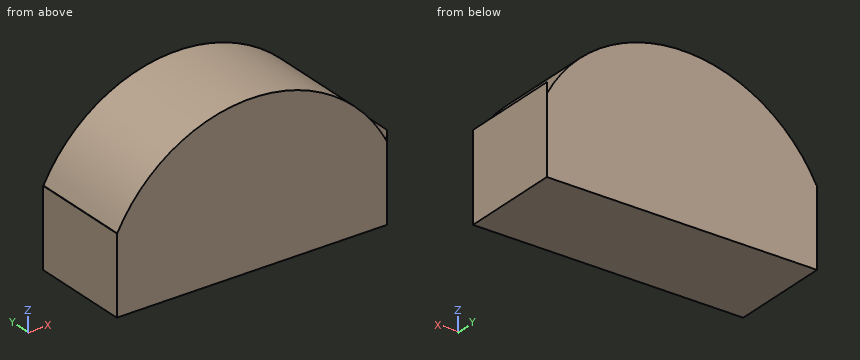
Solid Edge part; units mm, degrees
sketch "Sketch1" plane through (0, 0, 0) normal (0, 0, 1) x (1, 0, 0)
  line L0 (-40, -15) -> (40, -15)
  line L1 (40, -15) -> (40, 15)
  line L2 (40, 15) -> (-40, 15)
  line L3 (-40, 15) -> (-40, -15)
extrude "Protrusion1" add sketch "Sketch1" against normal blind 47
sketch "Sketch2" plane through (0, -15, -23.5) normal (0, -1, 0) x (1, 0, 0)
  arc A0 (39.8736, -0.641) -> (-39.8736, -0.641) centre (0, -21.5) ccw
  line L0 (-39.8736, -0.641) -> (-39.8736, 31.8802)
  line L1 (-39.8736, 31.8802) -> (41.2874, 31.8802)
  line L2 (41.2874, 31.8802) -> (39.8736, -0.641)
extrude "Recorte_Extrudado_3" cut sketch "Sketch2" against normal blind 30
sketch "Sketch3" plane through (0, -15, -23.5) normal (0, -1, 0) x (1, 0, 0)
  line L0 (-39.8736, -0.641) -> (-45.2071, -0.641)
  line L1 (-45.2071, -0.641) -> (-45.2071, 27.0459)
  line L2 (-45.2071, 27.0459) -> (-33.448, 27.0459)
  line L3 (-33.448, 27.0459) -> (-39.8736, -0.641)
extrude "Recorte_Extrudado_4" cut sketch "Sketch3" against normal blind 30
CAD build for the part. Positions are in the model's coordinates, mm. Round coordinates to 2 decimals unless told otherwise and drop trailing zeros. Order: outer loops, then holes, each group sorted by start corner. A loop starts at its lowest first (then second) coordinate and runs counter-clockwise, first axis right, second up. Notation, with made-up numbers: (-28.5, 19) -> (9.5, 19) arc R11 cw to (9.5, 33) -> close; hole circle Ø6 at (74, 55.25). An arc over 180 degrees is marked (long way). Write item = value, one per line. Start each with the question number.
(1) Pin check, flat tips, straight feed: P1, Ø8, axis at y = 5, z = -21, coming from the -X side; P2, Ø1, axis at x = 3, y = 5.5, coming from the +Z side; P3, Ø8, axis at y = 11.5, z = -9, coming from the -X side; P4, Ø2, axis at y = 3.5, z = -7.5, coming from the -X side. Stop position of each tip, or through.
(2) Cut at C-C, the plane x = 31. List the corners of the cut face in (y, z), then the cut area to 3 significant figures.
(3) Cut at B-B, the plane z = -9. List the corners of the cut face in (x, y).
(4) Probe line 1 (Z direction, x = 7.5, y = 5); line 2 (Z direction, x = 10, y = -3); line 3 (X direction, y = -13, z = -10). List the from-to ranges inside material, lowest first. Write a range as [from, to].
Model answer:
q1.P1 = -40
q1.P2 = -0.07
q1.P3 = -31.64
q1.P4 = -26.32
q2.outline = (-15, -47) -> (15, -47) -> (15, -12.38) -> (-15, -12.38) -> close
q2.area = 1,040 mm2
q3.outline = (-27, -15) -> (27, -15) -> (27, 15) -> (-27, 15) -> close
q4.line_1 = [-47, -0.63]
q4.line_2 = [-47, -1.13]
q4.line_3 = [-28.28, 28.28]
